For this review, take the finished solid that the model builds, in its own axes (mm). A direction names the side the tool comes from. Coordinates: 2 decimals unless noted, no trailing zeros. Loops run counter-clockwise (first coordinate to the right, second up) from the corner with the lowest first, then second, coordinate; pieces in that order, holes last. Notation, with made-up numbers: (39, 37.25) -> (49, 37.25) arc R8 ccw to (49, 51.25) -> close; hole circle Ø5 at (-24.75, -33). An arc over 180 degrees is marked (long way). Answer in a Markdown table with one row per item.
from build123d import *

# Parameters (mm, degrees)
F0_W     = 13
F0_H     = 1
F2_R     = 4.1
F3_DEPTH = 2.8
F4_R     = 3.225
F5_DEPTH = 2.1
F6_R     = 0.875
F7_DEPTH = 5.901
F8_DEPTH = 1
F9_SIZE  = 0.5
F10_SIZE = 2


with BuildPart() as f1:
    # F0 (on Front) → F1 (revolve)
    with BuildSketch(Plane.XZ):
        with Locations((6.5, 0.5)):
            Rectangle(F0_W, F0_H)
    revolve(axis=Axis((0, 0, 1.7087265151), (0, 0, 1)))

    # F2 (on face) → F3 (join)
    with BuildSketch(Plane.XY.offset(1)):
        Circle(F2_R)
    extrude(amount=F3_DEPTH)

    # F4 (on face) → F5 (join)
    with BuildSketch(Plane.XY.offset(3.8)):
        Circle(F4_R)
    extrude(amount=F5_DEPTH)

    # F6 (on face) → F7 (cut, through all)
    with BuildSketch(Plane.XY.offset(5.9)):
        Circle(F6_R)
    extrude(amount=-F7_DEPTH, mode=Mode.SUBTRACT)

    # F8 (add): a face of the model
    f8_faces = [f1.faces().sort_by_distance(p)[0] for p in [
        (-12.6323044738, 0, 0),
    ]]
    extrude(f8_faces, amount=F8_DEPTH)

    # F9
    f9_edges = [f1.edges().sort_by_distance(p)[0] for p in [
        (-13, 0, -1),
        (-13, 0, 1),
        (-3.225, 0, 5.9),
    ]]
    chamfer(f9_edges, length=F9_SIZE)

    # F10
    f10_edges = [f1.edges().sort_by_distance(p)[0] for p in [
        (-0.875, 0, -1),
    ]]
    chamfer(f10_edges, length=F10_SIZE)


solid = f1.part
Item 1: For L1, parallel to Y at x = 0, z = 2 (3 decimals); L2, parallel to Z at x = 2.25, y = -5; L3, parallel to Y at x = 1.25, z = 1.25, list the stretches that pass through material, from the lowest coordinate up.
Worked answers:
| item | result |
|---|---|
| L1 | -4.1 to -0.875, 0.875 to 4.1 |
| L2 | -1 to 1 |
| L3 | -3.9 to 3.9 |
Item 2: The part is to be moulded in two halves that separate along Y. For faces 1 (the flat face through (0, -5, 1)), 2 (the cylindrical face through (0.808, -0.335, 3.484)), 3 (the cylindrical face through (-0.7, -3.15, 4.59)), say which applies: +Y half, -Y half, draft (parallel to the pull), parting line (faces both ways), or undercut.
Worked answers:
| item | result |
|---|---|
| face 1 | draft |
| face 2 | undercut |
| face 3 | parting line |
Item 3: Take a section at C-C, the plane z = 3.25. State the section outline as (x, y) points (3 decimals), and give its area (3 significant figures).
Worked answers:
| item | result |
|---|---|
| outline | circle Ø8.2 at (0, 0); hole circle Ø1.75 at (0, 0) |
| area | 50.4 mm² |
Item 4: Insertion check: pin 1 (2 mm diameter, centred on x = 0, y = 7.5, fed in from +Z). The pin has a flat end and moves straight along its axis. Give the tip position at first contact, or say it passes through.
Worked answers:
| item | result |
|---|---|
| pin 1 | z = 1 |
Item 5: Take a section at A-A, the plane x = 0. State the section outline as (y, z) points (3 decimals).
Worked answers:
| item | result |
|---|---|
| outline | (-13, -0.5) -> (-12.5, -1) -> (-2.875, -1) -> (-0.875, 1) -> (-0.875, 5.9) -> (-2.725, 5.9) -> (-3.225, 5.4) -> (-3.225, 3.8) -> (-4.1, 3.8) -> (-4.1, 1) -> (-12.5, 1) -> (-13, 0.5) -> close; (0.875, 1) -> (2.875, -1) -> (12.5, -1) -> (13, -0.5) -> (13, 0.5) -> (12.5, 1) -> (4.1, 1) -> (4.1, 3.8) -> (3.225, 3.8) -> (3.225, 5.4) -> (2.725, 5.9) -> (0.875, 5.9) -> close |
Item 6: For faces 4 (the flat face through (-1, 1, 5.9)), 5 (the flat face through (2, -3, 3.8)), list the 3-axis set-ups (+Z, -Z, +X, -X, +Y, -Y) from which the entire face can be reached by the end or side of a thin tool; tool diameter is ignored.
Worked answers:
| item | result |
|---|---|
| face 4 | +Z, +X, -X, +Y, -Y |
| face 5 | +Z |
